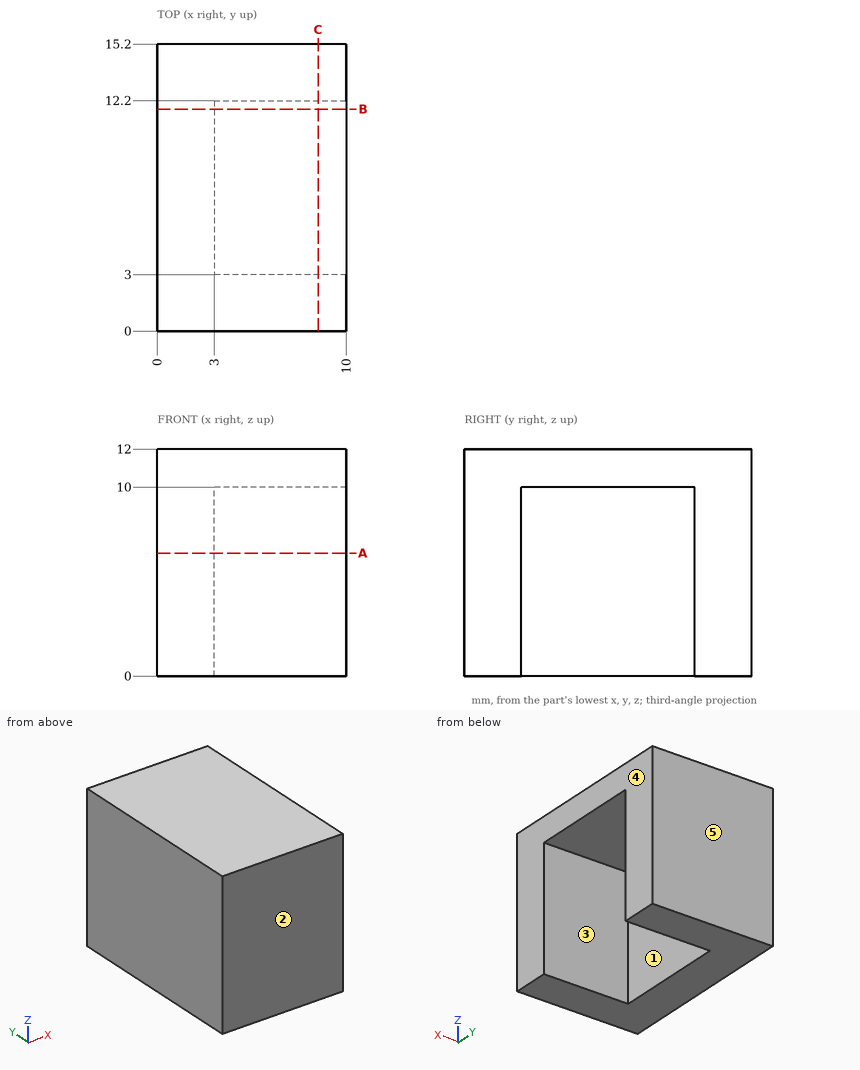
Here's the drawing with two shaded views (mm, measured from the low corner). I have some questions. A direction names the side the tool comes from. Round coordinates to 2 decimals unless told otherwise and drop trailing zeros. Order: outer loops, then holes, each group sorted by start corner. A loop starts at its lowest first (then second) coordinate and runs counter-clockwise, first axis right, second up. Notation, with made-up numbers: (29, 0) -> (73, 0) arc R25 cw to (73, 17) -> close; hole circle Ø4 at (50.25, -3.5). An arc over 180 degrees is marked (long way). Use a Markdown table: item, result. Add a question column.
(1) Suppose I cut it at C-C, the plane x = 8.5. Please give me the cut outline in (y, z).
(2) Suppose I cut it at A-A, the plane z = 6.5. Please give me the cut outline in (x, y).
(3) For pin 1 Ø1.5 at (y, z) = (5, 3.5) entering from +X, with a flat end and sliding along its axis, tell me the tip position at first contact or that it passes through.
(4) Suppose I cut it at B-B, the plane y = 11.75. Please give me the cut outline in (x, z), and give its area (3 significant figures).
(5) If we mould it in two halves opening along Y, with no side actions, what happens to the marked faces 3, 4 and 5? For each: released by +Y, released by -Y, zero draft, split by the parting line, or undercut.
(6) For the marked faces 1 and 2, which set-ups out of +Z, -Z, +X, -X, +Y, -Y let a thin tool reach every point of the face, with its end or its side?
(7) I need wall thicknesses on line 1 along Y through (x, z) = (9.5, 3.25); line 2 along X through (y, z) = (8.5, 4); line 3 along Z through (x, y) = (8, 10.5). Which ranges of each line are inside material? Lowest first, please.
Verdict:
| question | item | result |
|---|---|---|
| 1 | outline | (0, 0) -> (3, 0) -> (3, 10) -> (12.2, 10) -> (12.2, 0) -> (15.2, 0) -> (15.2, 12) -> (0, 12) -> close |
| 2 | outline | (0, 0) -> (10, 0) -> (10, 3) -> (3, 3) -> (3, 12.2) -> (10, 12.2) -> (10, 15.2) -> (0, 15.2) -> close |
| 3 | pin 1 | x = 3 |
| 4 | outline | (0, 0) -> (3, 0) -> (3, 10) -> (10, 10) -> (10, 12) -> (0, 12) -> close |
| 4 | area | 50.0 mm2 |
| 5 | face 3 | undercut |
| 5 | face 4 | zero draft |
| 5 | face 5 | released by +Y |
| 6 | face 1 | -Z, +X |
| 6 | face 2 | +Z, -Z, +X, -X, -Y |
| 7 | line 1 | 0 to 3, 12.2 to 15.2 |
| 7 | line 2 | 0 to 3 |
| 7 | line 3 | 10 to 12 |
